Autodesk Inventor part; units mm, degrees
ref_plane "YZ Plane" through (0, 0, 0) normal (1, 0, 0) x (0, 1, 0)
ref_plane "XZ Plane" through (0, 0, 0) normal (0, 1, 0) x (-1, 0, 0)
ref_plane "XY Plane" through (0, 0, 0) normal (0, 0, 1) x (1, 0, 0)
sketch "Sketch1" plane through (0, 0, 0) normal (0, 1, 0) x (-1, 0, 0)
  line L0 (0, 0) -> (-80, 0)
  line L1 (-80, 0) -> (-80, -120)
  line L2 (-80, -120) -> (0, -120)
  line L3 (0, -120) -> (0, 0)
  line L4 (0, -120) -> (0, -123)
  line L5 (0, -123) -> (-20, -123)
  line L6 (-20, -123) -> (-20, -120)
  line L7 (-40, -123) -> (-60, -123)
  line L8 (-60, -123) -> (-60, -120)
  line L9 (-40, -120) -> (-40, -123)
  line L10 (-80, 0) -> (-80, 3)
  line L11 (-80, 3) -> (-60, 3)
  line L12 (-60, 3) -> (-60, 0)
  line L13 (-40, 3) -> (-20, 3)
  line L14 (-40, 0) -> (-40, 3)
  line L15 (-20, 3) -> (-20, 0)
  line L16 (0, 0) -> (3, 0)
  line L17 (3, 0) -> (3, -20)
  line L18 (3, -20) -> (0, -20)
  line L19 (3, -60) -> (0, -60)
  line L20 (3, -40) -> (3, -60)
  line L21 (0, -40) -> (3, -40)
  line L22 (3, -100) -> (0, -100)
  line L23 (3, -80) -> (3, -100)
  line L24 (0, -80) -> (3, -80)
  line L25 (-80, -120) -> (-83, -120)
  line L26 (-83, -120) -> (-83, -100)
  line L27 (-83, -100) -> (-80, -100)
  line L28 (-83, -60) -> (-80, -60)
  line L29 (-83, -80) -> (-83, -60)
  line L30 (-80, -80) -> (-83, -80)
  line L31 (-83, -20) -> (-80, -20)
  line L32 (-83, -40) -> (-83, -20)
  line L33 (-80, -40) -> (-83, -40)
  line L34 (0, -20) -> (0, -40)
  line L35 (0, -60) -> (0, -80)
  line L36 (0, -100) -> (0, -123)
  line L37 (-20, -120) -> (-40, -120)
  line L38 (-60, -120) -> (-83, -120)
  line L39 (-80, -100) -> (-80, -80)
  line L40 (-80, -60) -> (-80, -40)
  line L41 (-80, -20) -> (-80, 3)
  line L42 (-60, 0) -> (-40, 0)
  line L43 (-20, 0) -> (3, 0)
  line L44 (-80, 3) -> (-83, 3)
  line L45 (-83, 3) -> (-83, 0)
  line L46 (-83, 0) -> (-80, 0)
  line L47 (3, 0) -> (3, 3)
  line L48 (3, 3) -> (0, 3)
  line L49 (0, 3) -> (0, 0)
  line L50 (0, -120) -> (3, -120)
  line L51 (3, -120) -> (3, -123)
  line L52 (3, -123) -> (0, -123)
  line L53 (-80, -120) -> (-80, -123)
  line L54 (-80, -123) -> (-83, -123)
  line L55 (-83, -123) -> (-83, -120)
  dimension "d0" = 120
  dimension "d1" = 80
  dimension "d2" = 3
  dimension "d3" = 20
  dimension "d13" = 40
  dimension "d18" = 3
  dimension "d19" = 20
  dimension "d22" = 40
  dimension "d27" = 3
  dimension "d28" = 20
  dimension "d31" = 40
  dimension "d36" = 3
  dimension "d37" = 20
  dimension "d40" = 40
  dimension "d47" = 3
  dimension "d48" = 3
  dimension "d49" = 3
extrude "Extrusion3" add sketch "Sketch1" along normal blind 3
sketch "Sketch2" plane through (0, 3, 0) normal (0, 1, 0) x (1, 0, 0)
  line L0 (10, 10) -> (10, 40) construction
  line L1 (11.5, 10) -> (11.5, 40)
  line L2 (8.5, 40) -> (8.5, 10)
  arc A0 (8.5, 10) -> (11.5, 10) centre (10, 10) ccw
  arc A1 (11.5, 40) -> (8.5, 40) centre (10, 40) ccw
  line L3 (0, 40) -> (0, 20)
  line L4 (0, 0) -> (20, 0)
  point P0 (10, 25)
  dimension "d50" = 30
  dimension "d51" = 3
  dimension "d52" = 10
  dimension "d53" = 10
extrude "Extrusion4" cut sketch "Sketch2" against normal up to next
pattern_linear "Rectangular Pattern2" count 2 spacing 40 along (0, 0, -1) of "Extrusion4"
pattern_linear "Rectangular Pattern3" count 6 spacing 6 along (1, 0, 0) of "Extrusion4", "Rectangular Pattern2"
properties part number "ControlBoxTop" material "Wood (Birch)"
Can you work these out from the model? Positions are in its coordinate system, mm. A direction names the side the tool comes from. Coordinates: 2 decimals unless noted, no trailing zeros. Loops run counter-clockwise (first coordinate to the right, second up) from the corner with the lowest first, then second, coordinate; pieces in that order, holes last. Notation, with made-up numbers: (-32.5, 36) - (-7.5, 36) arc R26 cw to (-7.5, 51) - close; hole circle Ø5 at (-16.75, 32.25). An arc over 180 degrees is marked (long way). Use a Markdown table: item, result.
Item 1: I want a section at C-C on y = 2.05. Give the number of separate pieces and of enclosed holes in the cut face, and give its area (3 significant figures).
Numbers:
| item | result |
|---|---|
| separate pieces | 1 |
| enclosed holes | 12 |
| area | 9,070 mm2 |
Item 2: I want a section at A-A on z = -63. Please give me the cut outline in (x, y), and give its area (3 significant figures).
Numbers:
| item | result |
|---|---|
| outline | (0, 0) - (8.5, 0) - (8.5, 3) - (0, 3) - close; (11.5, 0) - (14.5, 0) - (14.5, 3) - (11.5, 3) - close; (17.5, 0) - (20.5, 0) - (20.5, 3) - (17.5, 3) - close; (23.5, 0) - (26.5, 0) - (26.5, 3) - (23.5, 3) - close; (29.5, 0) - (32.5, 0) - (32.5, 3) - (29.5, 3) - close; (35.5, 0) - (38.5, 0) - (38.5, 3) - (35.5, 3) - close; (41.5, 0) - (83, 0) - (83, 3) - (41.5, 3) - close |
| area | 195 mm2 |
Item 3: For faces 1 (the face through (20, 1, 2)), 2 (the face through (0, 1, -110)), 3 (the face through (80, 1, -90)), 4 (the face through (26.5, 2, -25)), which set-ups out of +Z, -Z, +X, -X, +Y, -Y let a thin tool reach every point of the face, with its end or its side?
Numbers:
| item | result |
|---|---|
| face 1 | +Z, +Y, -Y |
| face 2 | -X, +Y, -Y |
| face 3 | +X, +Y, -Y |
| face 4 | +Y, -Y |
Item 4: We'd pull the mould along Z, two halves only. Please class faces 5 (the face through (10, 1, 0)), 6 (the face through (40, 1, 1)), 7 (the face through (70, 1, -120)), 8 (the face through (-2, 1, -20)): released by +Z, released by -Z, zero draft, split by the parting line, or undercut.
Numbers:
| item | result |
|---|---|
| face 5 | released by +Z |
| face 6 | zero draft |
| face 7 | released by -Z |
| face 8 | undercut |
Item 5: I want a section at B-B on x = 28. Please give me the cut outline in (y, z).
Numbers:
| item | result |
|---|---|
| outline | (0, -120) - (3, -120) - (3, -81.5) - (0, -81.5) - close; (0, -48.5) - (3, -48.5) - (3, -41.5) - (0, -41.5) - close; (0, -8.5) - (3, -8.5) - (3, 3) - (0, 3) - close |
Item 6: If I drill on probe 1 along Z at (x, y) = (64, 2.7); probe 2 along X at (y, z) = (2.8, -104); probe 3 along X at (y, z) = (0.35, -86.5), over which ranges is the centre line in solid material (lowest first)? Write a range as from..to.
Numbers:
| item | result |
|---|---|
| probe 1 | z = -120..3 |
| probe 2 | x = 0..83 |
| probe 3 | x = -3..80 |
Item 7: Will these pins go through, and if not, where does the flat tip stop? pin 1 (1.5 mm diameter, centred on y = 2, z = -110.5, fed in from -X); pin 2 (1.5 mm diameter, centred on x = 11.5, y = 2, fed in from +Z).
Numbers:
| item | result |
|---|---|
| pin 1 | stops at x = 0 |
| pin 2 | stops at z = 0 |
Item 8: I want a section at D-D on x = 57.5. Please give me the cut outline in (y, z).
Numbers:
| item | result |
|---|---|
| outline | (0, -123) - (3, -123) - (3, 0) - (0, 0) - close |
